from build123d import *

# Parameters (mm, degrees)
EXTRUDE_THIN1_DEPTH = 2.5


with BuildPart() as part:
    # Sketch1 → Extrude-Thin1 (new body, symmetric)
    with BuildSketch(Plane.XY):
        with BuildLine():
            Line((-248, -54.5), (-30.32, -54.5))
            ThreePointArc((-30.32, -54.5), (-22.941113788, -51.949709478), (-18.71173445, -45.387370423))
            Line((-18.71173445, -45.387370423), (-7.188382014, 1.75703273))
            ThreePointArc((-7.188382014, 1.75703273), (0, 7.4), (7.188382014, 1.75703273))
            Line((7.188382014, 1.75703273), (18.71173445, -45.387370423))
            ThreePointArc((18.71173445, -45.387370423), (22.941113788, -51.949709478), (30.32, -54.5))
            Line((30.32, -54.5), (248, -54.5))
            Line((248, -54.5), (248, -55.8))
            Line((248, -55.8), (30.32, -55.8))
            ThreePointArc((30.32, -55.8), (22.138389765, -52.972272016), (17.448910582, -45.696038335))
            Line((17.448910582, -45.696038335), (5.925558147, 1.448364818))
            ThreePointArc((5.925558147, 1.448364818), (0, 6.1), (-5.925558147, 1.448364818))
            Line((-5.925558147, 1.448364818), (-17.448910582, -45.696038335))
            ThreePointArc((-17.448910582, -45.696038335), (-22.138389765, -52.972272016), (-30.32, -55.8))
            Line((-30.32, -55.8), (-248, -55.8))
            Line((-248, -55.8), (-248, -54.5))
        make_face()
    extrude(amount=EXTRUDE_THIN1_DEPTH, both=True)


solid = part.part
Model file for the job. Use its own axes, mm. A direction names the side the tool comes from. Give positions to 0.01 mm unless a question says otherwise; leave off trailing zeros. Order: outer loops, then holes, each group sorted by start corner. A loop starts at its lowest first (then second) coordinate and runs counter-clockwise, first axis right, second up. Notation, with made-up numbers: (65.5, 62) - (102.5, 62) arc R34 cw to (102.5, 96) - close; hole circle Ø5 at (21, 81.5). An arc over 180 degrees is marked (long way). One line per item, written item: value.
Item 1: Slice it at C-C (x = -85). List the corners of the cut face in (y, z), then the cut area to 3 significant figures.
Response values:
outline: (-55.8, -2.5) - (-54.5, -2.5) - (-54.5, 2.5) - (-55.8, 2.5) - close
area: 6.50 mm2
Item 2: Slice it at A-A (z = -0.8). List the corners of the cut face in (x, y), then the cut area to 3 significant figures.
Response values:
outline: (-248, -55.8) - (-30.32, -55.8) arc R13.25 ccw to (-17.45, -45.7) - (-5.93, 1.45) arc R6.1 cw to (5.93, 1.45) - (17.45, -45.7) arc R13.25 ccw to (30.32, -55.8) - (248, -55.8) - (248, -54.5) - (30.32, -54.5) arc R11.95 cw to (18.71, -45.39) - (7.19, 1.76) arc R7.4 ccw to (-7.19, 1.76) - (-18.71, -45.39) arc R11.95 cw to (-30.32, -54.5) - (-248, -54.5) - close
area: 759 mm2
Item 3: Wall check: line 1 (X direction, y = -45.5, z = 0.15); line 2 (Y direction, x = 120.5, z = -2.25); line 3 (X direction, y = -38, z = -0.7). Give the ranges that are in metal, low to high.
Response values:
line 1: -18.74 to -17.4, 17.4 to 18.74
line 2: -55.8 to -54.5
line 3: -16.91 to -15.57, 15.57 to 16.91
Item 4: Two-plate mould, pull along X, no slides. Class faces 3 (the cylindrical face through (22.24, -53.05, 0.04)), 4 (the cylindrical face through (-23.03, -52.02, 0.04)), 5 (the cylindrical face through (22.85, -51.88, 0.04)): released by +X, released by -X, zero draft, split by the parting line, or undercut.
Response values:
face 3: undercut
face 4: released by -X
face 5: released by +X
Item 5: Pin check, flat tip, straight feed: pin 1 Ø2.5 at (x, z) = (-99, 1) entering from +Y. Stop position of the tip, or through.
Response values:
pin 1: y = -54.5
Item 6: Tool access for faces 1 (the flat face through (-11.607, -21.794, 0.035)), 2 (the flat face through (-13.03, -22.15, 0.04)): list every direction of +Z, -Z, +X, -X, +Y, -Y with a clear straight run to the whole face (end or side of a thin tool).
Response values:
face 1: +Z, -Z, -Y
face 2: +Z, -Z, -X, +Y
Item 7: Slice it at D-D (x = 25). List the corners of the cut face in (y, z).
Response values:
outline: (-54.69, -2.5) - (-53.25, -2.5) - (-53.25, 2.5) - (-54.69, 2.5) - close
Item 8: Slice it at B-B (y = -37). List the corners of the cut face in (x, z), then the cut area to 3 significant figures.
Response values:
outline: (-16.66, -2.5) - (-15.32, -2.5) - (-15.32, 2.5) - (-16.66, 2.5) - close; (15.32, -2.5) - (16.66, -2.5) - (16.66, 2.5) - (15.32, 2.5) - close
area: 13.4 mm2
